Work out the finished part from the listing and answer in its coordinate system (mm). A direction names the side the tool comes from. Give positions to 0.01 mm unless a question says otherwise; leave off trailing zeros. Loops run counter-clockwise (first coordinate to the right, second up) from the corner with the lowest first, then second, coordinate; pieces in that order, holes last. Notation, with made-up numbers: M -11.75,-21 L 28.25,-21 A16 cw 28.25,7 Z; hole C 24,74 d8. An arc over 180 degrees is marked long. Write item = value, one per line. Start each with the question number.
1. Section A-A on z = 55 is taken. Determine the outline of the cut face in (x, y).
2. Section C-C on y = 109.5 is taken. Determine the outline of the cut face in (x, z), plus the area to 3 significant figures.
3. Flat-ended cylindrical pins translate along their axes: pin 1 Ø10 at (x, y) = (-14.5, -117) entering from +Z; pin 2 Ø2 at (x, z) = (-82, 34.5) entering from +Y. Find the tip coordinate at first contact, or state that the pin passes through.
4. Section B-B on x = 146 is taken. Determine the outline of the cut face in (y, z), plus the area to 3 significant figures.
5. For faces 1 (the face through (-3, -130, 35)), 2 (the face through (-3, 150, 5)), determine the directions among +Z, -Z, +X, -X, +Y, -Y from which every point of the face is accessible in a straight line to the end or side of a thin tool.
6. Consider L1, parallel to X at y = -100, z = 5.25; L2, parallel to Y at x = -200, z = 2; L3, parallel to Y at x = -171, z = 56. Determine where each line is inside the solid, lowest interval first. Write a range as [from, to].
Autodesk Inventor part; units mm, degrees
ref_plane "YZ Plane" through (0, 0, 0) normal (1, 0, 0) x (0, 1, 0)
ref_plane "XZ Plane" through (0, 0, 0) normal (0, 1, 0) x (-1, 0, 0)
ref_plane "XY Plane" through (0, 0, 0) normal (0, 0, 1) x (1, 0, 0)
sketch "Sketch1" plane through (0, 0, 0) normal (0, 0, 1) x (1, 0, 0)
  line L0 (250, -150) -> (-250, -150)
  line L1 (-250, -150) -> (-250, 150)
  line L2 (-250, 150) -> (250, 150)
  line L3 (250, 150) -> (250, -150)
  line L4 (250, -150) -> (-250, 150) construction
  line L5 (-250, -150) -> (250, 150) construction
  point P0 (0, 0)
  dimension "d0" = 500
  dimension "d1" = 300
extrude "Extrusion1" add sketch "Sketch1" along normal blind 10
sketch "Sketch2" plane through (0, 0, 10) normal (0, 0, 1) x (1, 0, 0)
  line L0 (-250, 150) -> (-250, -150)
  line L1 (-250, -150) -> (250, -150)
  line L2 (-250, -130) -> (250, -130)
  line L3 (250, -130) -> (250, -150)
  line L4 (250, -150) -> (-250, -150)
  line L5 (-250, -150) -> (-250, -130)
  point P0 (0, 0)
  dimension "d6" = 20
extrude "Extrusion2" add sketch "Sketch2" along normal blind 50
sketch "Sketch3" plane through (0, 0, 0) normal (0, 0, -1) x (-1, 0, 0)
  line L0 (-250, -150) -> (-250, 150)
  line L1 (-250, 150) -> (250, 150)
  line L2 (250, 150) -> (250, -150)
  line L3 (250, -150) -> (-250, -150)
  point P0 (0, 0)
  point P1 (-200, 100)
  point P2 (200, 100)
  point P3 (-200, -100)
  point P4 (200, -100)
  dimension "d7" = 50
  dimension "d8" = 50
  dimension "d9" = 50
  dimension "d10" = 50
  dimension "d11" = 50
  dimension "d12" = 50
  dimension "d13" = 50
  dimension "d14" = 50
hole "Hole1" at (200, 100, 0) at (-200, 100, 0) at (200, -100, 0) at (-200, -100, 0) direction (0, 0, 1) diameter 5 end through all
Verdict:
q1.outline = M -250,-150 L 250,-150 L 250,-130 L -250,-130 Z
q2.outline = M -250,0 L 250,0 L 250,10 L -250,10 Z
q2.area = 5,000 mm2
q3.pin_1 = 10
q3.pin_2 = -130
q4.outline = M -150,0 L 150,0 L 150,10 L -130,10 L -130,60 L -150,60 Z
q4.area = 4,000 mm2
q5.face_1 = +Z, +X, -X, +Y
q5.face_2 = +Z, -Z, +X, -X, +Y
q6.L1 = [-250, -202.5], [-197.5, 197.5], [202.5, 250]
q6.L2 = [-150, -102.5], [-97.5, 97.5], [102.5, 150]
q6.L3 = [-150, -130]
